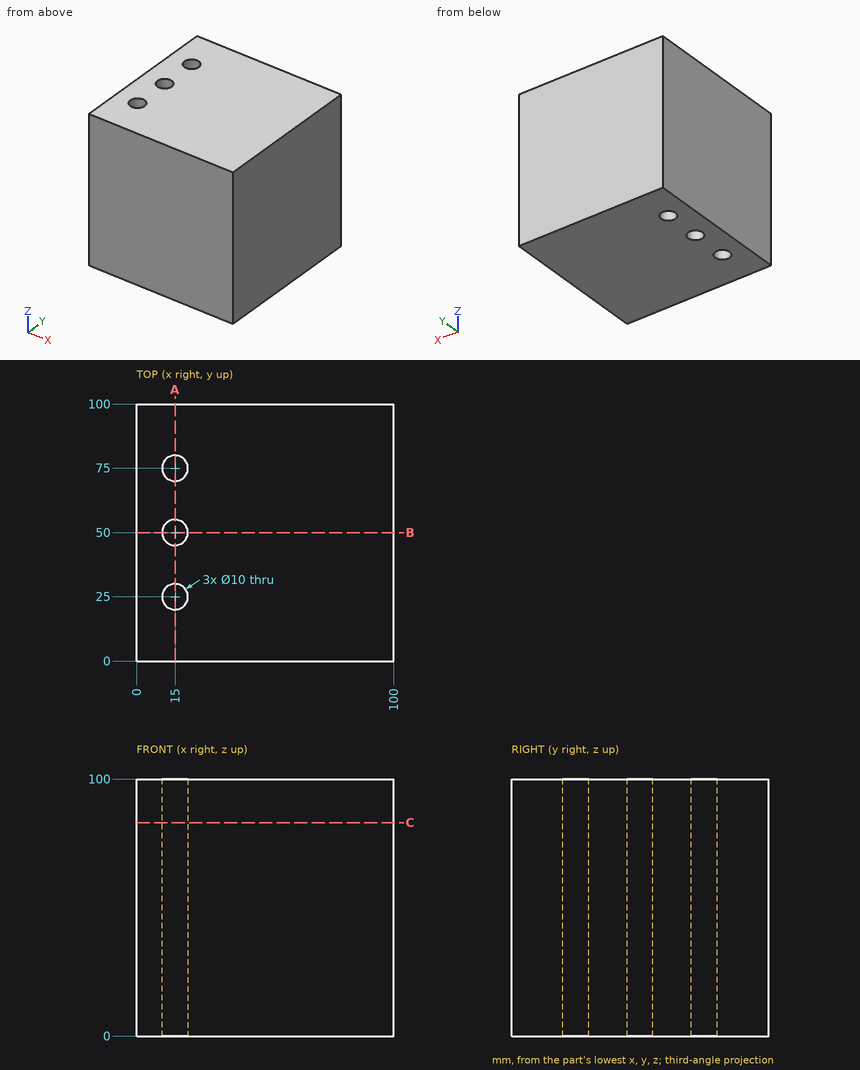
Check sheet for the drawn part. Datum: minimum x, y, z corner. Units: mm. Round coordinates to 2 decimals unless told otherwise and drop trailing zeros. Order: outer loops, then holes, each group sorted by start corner. A loop starts at its lowest first (then second) coordinate and runs counter-clockwise, first axis right, second up. Notation, with made-up numbers: (-37.5, 68.25) -> (11.5, 68.25) arc R13 cw to (11.5, 88.25) -> close; hole circle Ø4 at (71.25, 64). An arc over 180 degrees is marked (long way). Put each result on its own line as item: value. Start each with the question number.
(1) Section check C-C (z = 83). Enter the section's corners in (x, y).
(2) Depth check by flat-ended pin: pin 1 Ø8 at (x, y) = (15, 50) entering from +Z. Enter the tip coordinate at first touch or a pass-through.
(3) Section check B-B (y = 50). Enter the section's corners in (x, z), then the cut area to 3 significant figures.
(4) Material ranges on line 1 along Y through (x, z) = (15, 56); line 2 along Y through (x, z) = (10.5, 67.5); line 3 along X through (y, z) = (71, 79), recorded low to high.
(5) Section check A-A (x = 15). Enter the section's corners in (y, z), then the cut area to 3 significant figures.
Completed:
1. outline: (0, 0) -> (100, 0) -> (100, 100) -> (0, 100) -> close; hole circle Ø10 at (15, 25); hole circle Ø10 at (15, 50); hole circle Ø10 at (15, 75)
2. pin 1: passes through
3. outline: (0, 0) -> (10, 0) -> (10, 100) -> (0, 100) -> close; (20, 0) -> (100, 0) -> (100, 100) -> (20, 100) -> close
3. area: 9,000 mm2
4. line 1: y = 0 to 20, 30 to 45, 55 to 70, 80 to 100
4. line 2: y = 0 to 22.82, 27.18 to 47.82, 52.18 to 72.82, 77.18 to 100
4. line 3: x = 0 to 12, 18 to 100
5. outline: (0, 0) -> (20, 0) -> (20, 100) -> (0, 100) -> close; (30, 0) -> (45, 0) -> (45, 100) -> (30, 100) -> close; (55, 0) -> (70, 0) -> (70, 100) -> (55, 100) -> close; (80, 0) -> (100, 0) -> (100, 100) -> (80, 100) -> close
5. area: 7,000 mm2
